Part model, mm, in its own coordinate system. A direction names the side the tool comes from. Give positions to 0.01 mm unless a question says otherwise; leave off trailing zeros. Write each loop counter-clockwise with the first axis right and the second up, starting at its lowest first coordinate (ties: lowest second). Pieces come first, ordered by that corner, then holes. Notation, with made-up numbers: (88.5, 34.25) - (121.5, 34.25) arc R12 cw to (121.5, 38.25) - close; hole circle Ø9 at (-9, 70). An arc over 180 degrees is marked (long way). Answer as a JSON object with one key per item and string values. Group by question number.
```python
from build123d import *

# Parameters (mm, degrees)
BOSS_EXTRU_1_DEPTH      = 12.7
ESQUISSE2_R             = 3.175
ENL_V_MAT_EXTRU_1_DEPTH = 122.979516723
ENL_V_MAT_EXTRU_2_DEPTH = 122.979516723


with BuildPart() as part:
    # Esquisse1 → Boss.-Extru.1 (new body)
    with BuildSketch(Plane.XY):
        with BuildLine():
            Line((34.925, -88.9), (34.925, -75.458456647))
            ThreePointArc((34.925, -75.458456647), (41.275, -21.082), (47.625, -75.458456647))
            Line((47.625, -75.458456647), (47.625, -88.9))
            Line((47.625, -88.9), (82.55, -88.9))
            Line((82.55, -88.9), (82.55, 0))
            Line((82.55, 0), (0, 0))
            Line((0, 0), (0, -88.9))
            Line((0, -88.9), (34.925, -88.9))
        make_face()
    extrude(amount=BOSS_EXTRU_1_DEPTH)

    # Esquisse2 → Enlèv. mat.-Extru.1 (cut, through all)
    with BuildSketch(Plane(origin=(82.55, 0, 0), x_dir=(0, 0, -1), z_dir=(1, 0, 0))):
        with Locations(Location((-6.35, -82.55, 0), (0, 0, 90))):
            Circle(ESQUISSE2_R)
    extrude(amount=-ENL_V_MAT_EXTRU_1_DEPTH, mode=Mode.SUBTRACT)

    # Esquisse3 → Enlèv. mat.-Extru.2 (cut, through all)
    with BuildSketch(Plane.XY.offset(12.7)):
        Polygon((11.049, 0), (0, -21.684883475), (0, 0), align=None)
        Polygon((71.501, 0), (82.55, 0), (82.55, -21.684883475), align=None)
    extrude(amount=-ENL_V_MAT_EXTRU_2_DEPTH, mode=Mode.SUBTRACT)


solid = part.part
```
1) Saw through at D-D (y = -44.5). List the corners of the cut face in (x, z), and give its area (3 significant figures).
2) Drop flat-ended pins along their axis: P1, Ø2, axis at y = -12.5, z = 2.5, coming from the +X side; P2, Ø1.5, axis at y = -11.5, z = 5, coming from the -X side. Give the stop position or say it passes through.
3) Which spindle directions (+Z, -Z, +X, -X, +Y, -Y) get a long thin tool onto all of the face, cutting with end or side? Do faces 4 (the flat face through (42, 0, 6)), 5 (the flat face through (34.925, -79, 6)). Say none if no direction does.
4) Saw through at A-A (x = 52). List the corners of the cut face in (y, z) (3 decimals).
5) Drill centre lines: line 1 along X through (y, z) = (-48, 4.25); line 2 along X through (y, z) = (-84, 10) (3 decimals); line 3 along Z through (x, y) = (22, -82.55) (3 decimals). Where is each one in solid material? Low to high. Write a range as from..to.
6) Saw through at C-C (z = 6.35). List the corners of the cut face in (x, y) (3 decimals).
7) Saw through at B-B (y = -82.55). List the corners of the cut face in (x, z) (3 decimals), and give its area (3 significant figures).
8) Two-plate mould, pull along Y, no slides. Class faces 1 (the cylindrical face through (65.3, -80.8, 9)), 2 (the flat face through (0, -55, 6)), 3 (the flat face through (5.6, -10.69, 6.44)): +Y half, -Y half, draft (parallel to the pull), parting line (faces both ways), or undercut.
Checks:
{
 "1": {"outline": "(0, 0) - (14.03, 0) - (14.03, 12.7) - (0, 12.7) - close; (68.52, 0) - (82.55, 0) - (82.55, 12.7) - (68.52, 12.7) - close", "area": "356 mm2"},
 "2": {"P1": "x = 78.38", "P2": "x = 4.81"},
 "3": {"face 4": "+Z, -Z, +X, -X, +Y", "face 5": "+Z, -Z, -Y"},
 "4": {"outline": "(-88.9, 0) - (-74.027, 0) - (-74.027, 12.7) - (-88.9, 12.7) - close; (-23.255, 0) - (0, 0) - (0, 12.7) - (-23.255, 12.7) - close; hole circle Ø6.35 at (-82.55, 6.35)"},
 "5": {"line 1": "0..13.72, 68.83..82.55", "line 2": "0..34.925, 47.625..82.55", "line 3": "0..3.175, 9.525..12.7"},
 "6": {"outline": "(0, -88.9) - (34.925, -88.9) - (34.925, -85.725) - (0, -85.725) - close; (0, -79.375) - (34.925, -79.375) - (34.925, -75.458) arc R27.559 cw (long way) to (47.625, -75.458) - (47.625, -79.375) - (82.55, -79.375) - (82.55, -21.685) - (71.501, 0) - (11.049, 0) - (0, -21.685) - close; (47.625, -88.9) - (82.55, -88.9) - (82.55, -85.725) - (47.625, -85.725) - close"},
 "7": {"outline": "(0, 0) - (34.925, 0) - (34.925, 3.175) - (0, 3.175) - close; (0, 9.525) - (34.925, 9.525) - (34.925, 12.7) - (0, 12.7) - close; (47.625, 0) - (82.55, 0) - (82.55, 3.175) - (47.625, 3.175) - close; (47.625, 9.525) - (82.55, 9.525) - (82.55, 12.7) - (47.625, 12.7) - close", "area": "444 mm2"},
 "8": {"face 1": "undercut", "face 2": "draft", "face 3": "+Y half"}
}
